Study the drawing (mm; zero at the part's minimum x, y, z) and answer. Coordinates: 2 decimals unless noted, no trailing zeros. Loops run counter-clockwise (first coordinate to the right, second up) from the corner with the lowest first, then second, coordinate; pieces in that order, holes last. Notation, with made-up numbers: M 83,45 L 117,45 A13 cw 117,54 Z; hole C -3.5,49 d5. An arc over 180 degrees is marked long. Use one line per item in the form item = value. Start each with the question number.
1. The part is cut by section B-B (z = 2.5). Give the number of separate pieces and of enclosed holes in the cut face, plus the area to 3 significant figures.
2. Flat-ended cylindrical pins translate along their axes: pin 1 (4 mm diameter, centred on x = 30, y = 19.05, fed in from +Z) (3 decimals); pin 2 (6 mm diameter, centred on x = 50, y = 19.05, fed in from -Z). Find the tip coordinate at first contact, or state that the pin passes through.
3. The part is cut by section A-A (x = 50). Give the vertices of the cut face in (y, z), plus the area to 3 significant figures.
4. Find the intervals of material crossed by probe 1 along Y at (x, z) = (50, 4); probe 2 along X at (y, z) = (17, 5); probe 3 along Y at (x, z) = (230.95, 2.75), in increasing order. Write a range as [from, to].
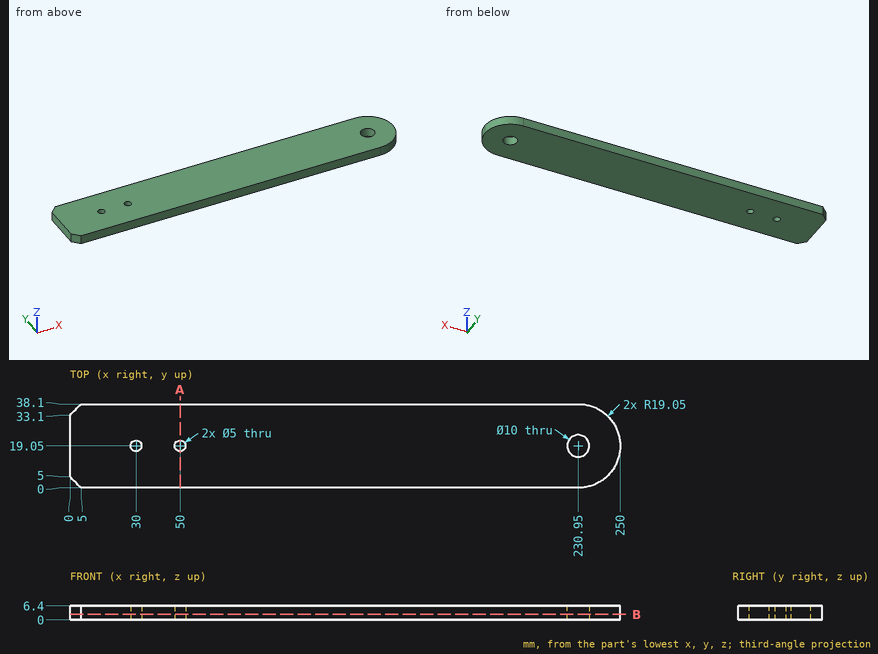
Computed values:
q1.separate_pieces = 1
q1.enclosed_holes = 3
q1.area = 9,230 mm²
q2.pin_1 = through
q2.pin_2 = 0
q3.outline = M 0,0 L 16.55,0 L 16.55,6.4 L 0,6.4 Z; M 21.55,0 L 38.1,0 L 38.1,6.4 L 21.55,6.4 Z
q3.area = 212 mm²
q4.probe_1 = [0, 16.55], [21.55, 38.1]
q4.probe_2 = [0, 28.57], [31.43, 48.57], [51.43, 226.39], [235.51, 249.89]
q4.probe_3 = [0, 14.05], [24.05, 38.1]
